```python
from build123d import *

# Parameters (mm, degrees)
EXTRUDE_1_DEPTH               = 12.7
SKETCH_2_R                    = 3.3782
CUT_EXTRUDE_1_DEPTH           = 184.601770144
SKETCH_5_R                    = 10.3125
CUT_EXTRUDE_4_DEPTH           = 7.95
SKETCH_6_R                    = 6.7435
CUT_EXTRUDE_5_DEPTH           = 184.601770144
SKETCH_7_R                    = 9.525
CUT_EXTRUDE_6_DEPTH           = 5.245104753
CUT_EXTRUDE_6_DRAFT           = -41
SKETCH_8_R                    = 4.9655
CUT_EXTRUDE_7_DEPTH           = 184.601770144
SKETCH_9_R                    = 2.0193
CUT_EXTRUDE_8_DEPTH           = 9.525
SKETCH_10_R                   = 2.0193
CUT_EXTRUDE_9_DEPTH           = 1.210313545
CUT_EXTRUDE_9_DRAFT           = -59
CUT_EXTRUDE_9_PROFILE_2_DEPTH = 1.210313545
CUT_EXTRUDE_9_PROFILE_2_DRAFT = -59
CUT_EXTRUDE_9_PROFILE_3_DEPTH = 1.210313545
CUT_EXTRUDE_9_PROFILE_3_DRAFT = -59
CUT_EXTRUDE_10_DEPTH          = 184.601770144
CHAMFER_1_SIZE                = 0.762


with BuildPart() as part:
    # 草图1 → 凸台-拉伸1 (new body)
    with BuildSketch(Plane.XY):
        with BuildLine():
            Line((6.35, 0), (146.05, 0))
            ThreePointArc((146.05, 0), (150.540128061, 1.859871939), (152.4, 6.35))
            Line((152.4, 6.35), (152.4, 95.25))
            ThreePointArc((152.4, 95.25), (150.540128061, 99.740128061), (146.05, 101.6))
            Line((146.05, 101.6), (6.35, 101.6))
            ThreePointArc((6.35, 101.6), (1.859871939, 99.740128061), (0, 95.25))
            Line((0, 95.25), (0, 6.35))
            ThreePointArc((0, 6.35), (1.859871939, 1.859871939), (6.35, 0))
        make_face()
    extrude(amount=EXTRUDE_1_DEPTH)

    # 草图2 → 切除-拉伸1 (cut, through all)
    with BuildSketch(Plane.XY.offset(12.7)):
        with Locations((9.525, 9.525)):
            Circle(SKETCH_2_R)
        with Locations((142.875, 9.525)):
            Circle(SKETCH_2_R)
        with Locations((9.525, 92.075)):
            Circle(SKETCH_2_R)
        with Locations((142.875, 92.075)):
            Circle(SKETCH_2_R)
    extrude(amount=-CUT_EXTRUDE_1_DEPTH, mode=Mode.SUBTRACT)

    # 草图5 → 切除-拉伸4 (cut)
    with BuildSketch(Plane.XY.offset(12.7)):
        with Locations((38.1, 50.8)):
            Circle(SKETCH_5_R)
    extrude(amount=-CUT_EXTRUDE_4_DEPTH, mode=Mode.SUBTRACT)

    # 草图6 → 切除-拉伸5 (cut, through all)
    with BuildSketch(Plane.XY.offset(12.7)):
        with Locations((38.1, 50.8)):
            Circle(SKETCH_6_R)
    extrude(amount=-CUT_EXTRUDE_5_DEPTH, mode=Mode.SUBTRACT)


with BuildPart() as cut_extrude_6_tool:
    # 草图7 → 切除-拉伸6 (with draft: the straight prism first)
    with BuildSketch(Plane.XY.offset(12.7)):
        with Locations((114.3, 50.8)):
            Circle(SKETCH_7_R)
    extrude(amount=-CUT_EXTRUDE_6_DEPTH)
    # 切除-拉伸6: the draft: its side faces are tilted about the plane it starts from
    cut_extrude_6_sides = [cut_extrude_6_tool.faces().sort_by_distance(p)[0] for p in [
        (104.775, 50.8, 10.077447624),
    ]]
    draft(cut_extrude_6_sides, Plane.XY.offset(12.7), CUT_EXTRUDE_6_DRAFT)


with BuildPart() as part_1:
    add(part.part)

    # 切除-拉伸6: cut by cut_extrude_6_tool
    add(cut_extrude_6_tool.part, mode=Mode.SUBTRACT)

    # 草图8 → 切除-拉伸7 (cut, through all)
    with BuildSketch(Plane.XY.offset(12.7)):
        with Locations((114.3, 50.8)):
            Circle(SKETCH_8_R)
    extrude(amount=-CUT_EXTRUDE_7_DEPTH, mode=Mode.SUBTRACT)

    # 草图9 → 切除-拉伸8 (cut)
    with BuildSketch(Plane.XY.offset(12.7)):
        with Locations((114.3, 66.675)):
            Circle(SKETCH_9_R)
        with Locations((100.551847, 42.8625)):
            Circle(SKETCH_9_R)
        with Locations((128.048153, 42.8625)):
            Circle(SKETCH_9_R)
    extrude(amount=-CUT_EXTRUDE_8_DEPTH, mode=Mode.SUBTRACT)


with BuildPart() as cut_extrude_9_tool:
    # 草图10 → 切除-拉伸9 (with draft: the straight prism first)
    with BuildSketch(Plane.XY.offset(3.175)):
        with Locations((114.3, 66.675)):
            Circle(SKETCH_10_R)
    extrude(amount=-CUT_EXTRUDE_9_DEPTH)
    # 切除-拉伸9: the draft: its side faces are tilted about the plane it starts from
    cut_extrude_9_sides = [cut_extrude_9_tool.faces().sort_by_distance(p)[0] for p in [
        (112.2807, 66.675, 2.569843228),
    ]]
    draft(cut_extrude_9_sides, Plane.XY.offset(3.175), CUT_EXTRUDE_9_DRAFT)


with BuildPart() as part_2:
    add(part_1.part)

    # 切除-拉伸9: cut by cut_extrude_9_tool
    add(cut_extrude_9_tool.part, mode=Mode.SUBTRACT)


with BuildPart() as cut_extrude_9_profile_2_tool:
    # 草图10 → 切除-拉伸9 profile 2 (with draft: the straight prism first)
    with BuildSketch(Plane.XY.offset(3.175)):
        with Locations((100.551847, 42.8625)):
            Circle(SKETCH_10_R)
    extrude(amount=-CUT_EXTRUDE_9_PROFILE_2_DEPTH)
    # 切除-拉伸9 profile 2: the draft: its side faces are tilted about the plane it starts from
    cut_extrude_9_profile_2_sides = [cut_extrude_9_profile_2_tool.faces().sort_by_distance(p)[0] for p in [
        (98.532547, 42.8625, 2.569843228),
    ]]
    draft(cut_extrude_9_profile_2_sides, Plane.XY.offset(3.175), CUT_EXTRUDE_9_PROFILE_2_DRAFT)


with BuildPart() as part_3:
    add(part_2.part)

    # 切除-拉伸9 profile 2: cut by cut_extrude_9_profile_2_tool
    add(cut_extrude_9_profile_2_tool.part, mode=Mode.SUBTRACT)


with BuildPart() as cut_extrude_9_profile_3_tool:
    # 草图10 → 切除-拉伸9 profile 3 (with draft: the straight prism first)
    with BuildSketch(Plane.XY.offset(3.175)):
        with Locations((128.048153, 42.8625)):
            Circle(SKETCH_10_R)
    extrude(amount=-CUT_EXTRUDE_9_PROFILE_3_DEPTH)
    # 切除-拉伸9 profile 3: the draft: its side faces are tilted about the plane it starts from
    cut_extrude_9_profile_3_sides = [cut_extrude_9_profile_3_tool.faces().sort_by_distance(p)[0] for p in [
        (126.028853, 42.8625, 2.569843228),
    ]]
    draft(cut_extrude_9_profile_3_sides, Plane.XY.offset(3.175), CUT_EXTRUDE_9_PROFILE_3_DRAFT)


with BuildPart() as part_4:
    add(part_3.part)

    # 切除-拉伸9 profile 3: cut by cut_extrude_9_profile_3_tool
    add(cut_extrude_9_profile_3_tool.part, mode=Mode.SUBTRACT)

    # 草图11 → 切除-拉伸10 (cut, through all)
    with BuildSketch(Plane.XY.offset(12.7)):
        with BuildLine():
            Line((63.5, 15.875), (88.9, 15.875))
            ThreePointArc((88.9, 15.875), (92.075, 19.05), (88.9, 22.225))
            Line((88.9, 22.225), (63.5, 22.225))
            ThreePointArc((63.5, 22.225), (60.325, 19.05), (63.5, 15.875))
        make_face()
    extrude(amount=-CUT_EXTRUDE_10_DEPTH, mode=Mode.SUBTRACT)

    # 倒角1
    chamfer_1_edges = [part_4.edges().sort_by_distance(p)[0] for p in [
        (150.540128061, 1.859871939, 12.7),
        (152.4, 50.8, 12.7),
        (150.540128061, 99.740128061, 12.7),
        (76.2, 101.6, 12.7),
        (1.859871939, 99.740128061, 12.7),
        (0, 50.8, 12.7),
        (1.859871939, 1.859871939, 12.7),
        (76.2, 0, 12.7),
    ]]
    chamfer(chamfer_1_edges, length=CHAMFER_1_SIZE)


solid = part_4.part
```
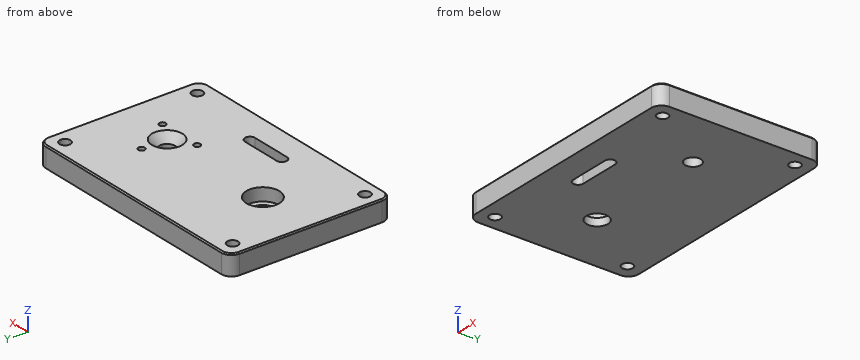
Source: CAD feature listing. Evaluate the final solid. Frame: model axes, mm. Round coordinates to 2 decimals unless told otherwise and drop trailing zeros. Order: outer loops, then holes, each group sorted by start corner. A loop starts at its lowest first (then second) coordinate and runs counter-clockwise, first axis right, second up. Notation, with made-up numbers: (-22, 15.5) -> (12, 15.5) arc R22 cw to (12, 25.5) -> close; hole circle Ø9 at (30, -27.5). An arc over 180 degrees is marked (long way). One line per item, written item: value. Start each with the question number.
Q1. Section query D-D (x = 78). Return the cut outline in (y, z) (3 decimals).
Q2. Section query C-C (x = 10.5). Return the cut outline in (y, z).
Q3. Material intervals for probe 1 along X at (y, z) = (10, 6.25); probe 2 along Y at (x, z) = (38, 3.75); probe 3 along X at (y, z) = (10.5, 3.5), sorted ascending.
Q4. Section query B-B (y = 19.05). Return the cut outline in (x, z) (3 decimals).
Q5. Section query A-A (y = 50.8). Give the number of separate pieces and of enclosed holes in the cut face, plus the area to 3 significant figures.
Findings below:
1. outline: (0, 0) -> (15.875, 0) -> (15.875, 12.7) -> (0.762, 12.7) -> (0, 11.938) -> close; (22.225, 0) -> (101.6, 0) -> (101.6, 11.938) -> (100.838, 12.7) -> (22.225, 12.7) -> close
2. outline: (0, 0) -> (6.29, 0) -> (6.29, 12.7) -> (0.76, 12.7) -> (0, 11.94) -> close; (12.76, 0) -> (88.84, 0) -> (88.84, 12.7) -> (12.76, 12.7) -> close; (95.31, 0) -> (101.6, 0) -> (101.6, 11.94) -> (100.84, 12.7) -> (95.31, 12.7) -> close
3. probe 1: 0 to 6.18, 12.87 to 139.53, 146.22 to 152.4
3. probe 2: 0 to 44.06, 57.54 to 101.6
3. probe 3: 0 to 6.29, 12.76 to 139.64, 146.11 to 152.4
4. outline: (0, 0) -> (60.325, 0) -> (60.325, 12.7) -> (0.762, 12.7) -> (0, 11.938) -> close; (92.075, 0) -> (152.4, 0) -> (152.4, 11.938) -> (151.638, 12.7) -> (92.075, 12.7) -> close
5. separate pieces: 3
5. enclosed holes: 0
5. area: 1,560 mm²
